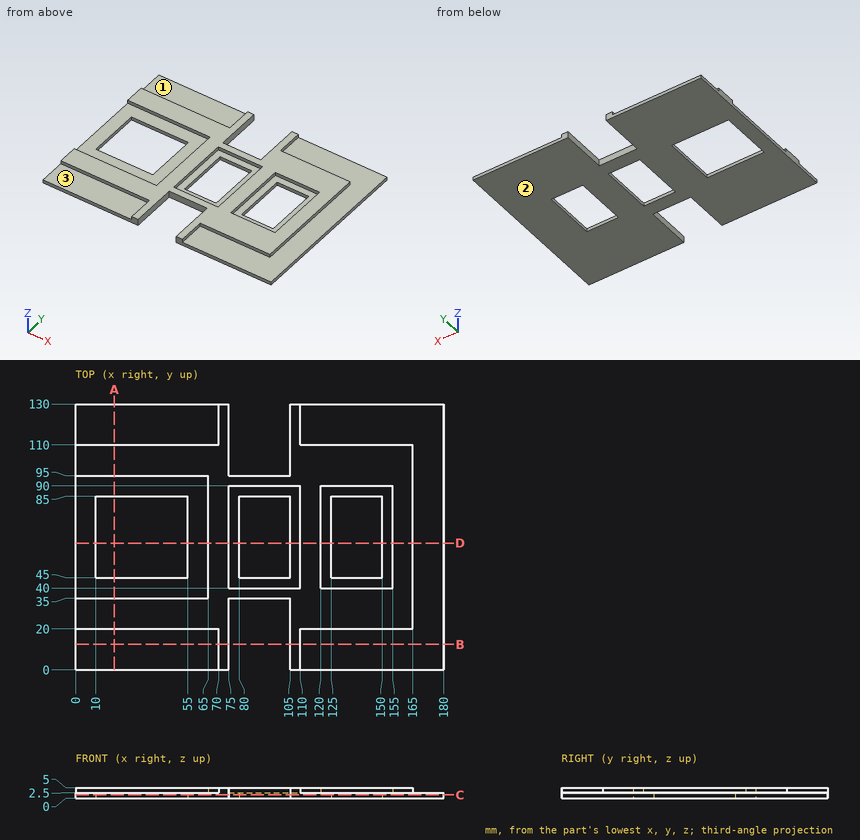
Print and shaded views of the part. All mm, measured from the part's lowest x, y and z. A direction names the side the tool comes from. Coordinates: 2 decimals unless noted, no trailing zeros. Loops run counter-clockwise (first coordinate to the right, second up) from the corner with the lowest first, then second, coordinate; pieces in that order, holes last. Notation, with made-up numbers: (44.25, -18.75) -> (85.25, -18.75) arc R15 cw to (85.25, -1.75) -> close; hole circle Ø3 at (-35.75, 6). An arc over 180 degrees is marked (long way). Use a Markdown table: item, result. Add a question column.
Item 1: Band-saw the part on C-C on z = 1.6. Write the cut outline in (x, y).
Item 2: Band-saw the part on A-A on x = 19. Write the cut outline in (y, z), plus the area to 3 significant figures.
Item 3: Probe probe 1 along X at (y, z) = (42.5, 3.35); probe 2 along X at (y, z) = (56.5, 1.6); probe 3 along X at (y, z) = (11, 4.6). List the from-to ranges inside material, lowest first.
Item 4: Flat gauge pins, fed straight in: P1, Ø0.8, axis at y = 53.5, z = 3.5, coming from the +X side; P2, Ø1.5, axis at x = 112, z = 3.5, coming from the +Y side; P3, Ø2.5, axis at x = 88.5, z = 2, coming from the +Y side. Where does each tip first touch, or does it go through?
Item 5: Band-saw the part on B-B on y = 12.5. Write the cut outline in (x, z).
Item 6: Band-saw the part on D-D on y = 62. Write the cut outline in (x, z), plus the area to 4 significant figures.
Item 7: Which spindle directions (+Z, -Z, +X, -X, +Y, -Y) get a long thin tool onto all of the face, cutting with end or side? Do the marked faces 1, 2 and 3. Say none if no direction does.
Geometry says:
| question | item | result |
|---|---|---|
| 1 | outline | (0, 0) -> (75, 0) -> (75, 35) -> (105, 35) -> (105, 0) -> (180, 0) -> (180, 130) -> (105, 130) -> (105, 95) -> (75, 95) -> (75, 130) -> (0, 130) -> close; hole (10, 45) -> (55, 45) -> (55, 85) -> (10, 85) -> close; hole (80, 45) -> (105, 45) -> (105, 85) -> (80, 85) -> close; hole (125, 45) -> (150, 45) -> (150, 85) -> (125, 85) -> close |
| 2 | outline | (0, 0) -> (45, 0) -> (45, 2.5) -> (35, 2.5) -> (35, 5) -> (20, 5) -> (20, 2.5) -> (0, 2.5) -> close; (85, 0) -> (130, 0) -> (130, 2.5) -> (110, 2.5) -> (110, 5) -> (95, 5) -> (95, 2.5) -> (85, 2.5) -> close |
| 2 | area | 300 mm² |
| 3 | probe 1 | 65 to 75, 110 to 120, 155 to 165 |
| 3 | probe 2 | 0 to 10, 55 to 80, 105 to 125, 150 to 180 |
| 3 | probe 3 | 70 to 75, 105 to 110 |
| 4 | P1 | x = 165 |
| 4 | P2 | y = 110 |
| 4 | P3 | y = 95 |
| 5 | outline | (0, 0) -> (75, 0) -> (75, 5) -> (70, 5) -> (70, 2.5) -> (0, 2.5) -> close; (105, 0) -> (180, 0) -> (180, 2.5) -> (110, 2.5) -> (110, 5) -> (105, 5) -> close |
| 6 | outline | (0, 0) -> (10, 0) -> (10, 2.5) -> (0, 2.5) -> close; (55, 0) -> (80, 0) -> (80, 2.5) -> (75, 2.5) -> (75, 5) -> (65, 5) -> (65, 2.5) -> (55, 2.5) -> close; (105, 0) -> (125, 0) -> (125, 2.5) -> (120, 2.5) -> (120, 5) -> (110, 5) -> (110, 2.5) -> (105, 2.5) -> close; (150, 0) -> (180, 0) -> (180, 2.5) -> (165, 2.5) -> (165, 5) -> (155, 5) -> (155, 2.5) -> (150, 2.5) -> close |
| 6 | area | 287.5 mm² |
| 7 | face 1 | +Z, -X, +Y |
| 7 | face 2 | -Z, +X, -X, +Y, -Y |
| 7 | face 3 | +Z, -X, -Y |
